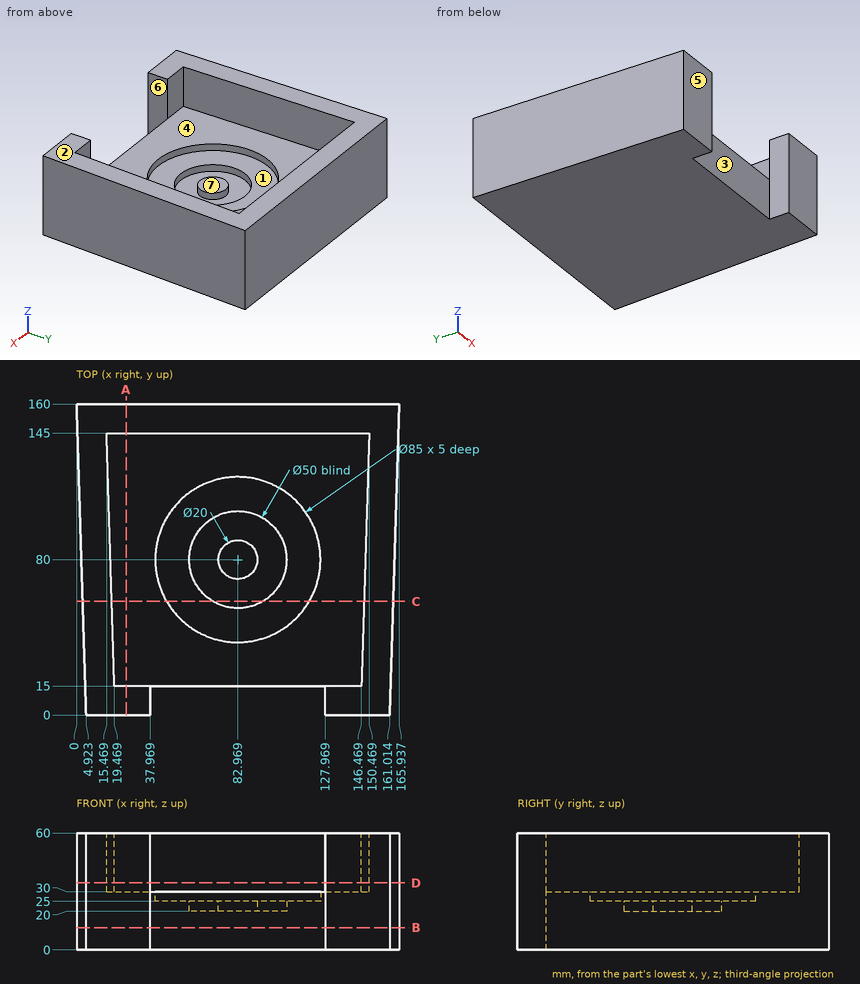
Can you work these out from the drawing? Everything is in mm from the part's minimum corner. A direction names the side the tool comes from. Coordinates: 2 decimals unless noted, no trailing zeros. Loops run counter-clockwise (first coordinate to the right, second up) from the corner with the lowest first, then second, coordinate; pieces in that order, holes last. Notation, with made-up numbers: (54, 83) -> (104, 83) arc R26 ccw to (104, 101) -> close; hole circle Ø6 at (0.5, 7). An arc over 180 degrees is marked (long way). Return JSON: item names as keys, results as strings.
1) If we section it at D-D, the plane z = 34.5: Write out the boundary of the cut face in (x, y), then the cut area to 3 significant figures.
Results below:
{"outline": "(0, 160) -> (4.92, 0) -> (37.97, 0) -> (37.97, 15) -> (19.47, 15) -> (15.47, 145) -> (150.47, 145) -> (146.47, 15) -> (127.97, 15) -> (127.97, 0) -> (161.01, 0) -> (165.94, 160) -> close", "area": "7,380 mm²"}
2) For the marked faces 1, 2 and 3, which set-ups out of +Z, -Z, +X, -X, +Y, -Y let a thin tool reach every point of the face, with its end or its side?
Results below:
{"face 1": "+Z", "face 2": "+Z, +X, -X, +Y, -Y", "face 3": "+Z, -Z, -Y"}
3) Will these pins go through, and if not, where does the flat tip stop? pin 1 (15 mm diameter, centred on x = 72.5, z = 46.5, fed in from -Y); pin 2 (4.5 mm diameter, centred on y = 8.5, z = 21.5, fed in from -X); pin 3 (3 mm diameter, centred on x = 69, y = 122.5, fed in from +Z).
Results below:
{"pin 1": "y = 145", "pin 2": "x = 4.59", "pin 3": "z = 30"}
4) I need wall thicknesses on line 1 (X direction, y = 80, z = 21) (1 decimal); line 2 (Z direction, x = 29.5, y = 106); line 3 (Z direction, x = 73, y = 94.5). Which ranges of each line are inside material? Lowest first, please. Write a range as from..to.
Results below:
{"line 1": "2.5..58, 73..93, 108..163.5", "line 2": "0..30", "line 3": "0..20"}
5) If we section it at C-C, the plane y = 58.5: Write out the boundary of the cut face in (x, z).
Results below:
{"outline": "(3.12, 0) -> (162.81, 0) -> (162.81, 60) -> (147.81, 60) -> (147.81, 30) -> (119.63, 30) -> (119.63, 25) -> (95.73, 25) -> (95.73, 20) -> (70.21, 20) -> (70.21, 25) -> (46.31, 25) -> (46.31, 30) -> (18.13, 30) -> (18.13, 60) -> (3.12, 60) -> close"}
6) If we section it at B-B, the plane z = 11.5: Write out the boundary of the cut face in (x, y).
Results below:
{"outline": "(0, 160) -> (4.92, 0) -> (37.97, 0) -> (37.97, 15) -> (127.97, 15) -> (127.97, 0) -> (161.01, 0) -> (165.94, 160) -> close"}
7) If we section it at A-A, the plane x = 25.5: Write out the boundary of the cut face in (y, z).
Results below:
{"outline": "(0, 0) -> (160, 0) -> (160, 60) -> (145, 60) -> (145, 30) -> (15, 30) -> (15, 60) -> (0, 60) -> close"}
8) Thinking about a two-plate mould opening in Y: for the marked faces 4, 5, 6 and 7, which applies, +Y half, -Y half, draft (parallel to the pull), parting line (faces both ways), or undercut?
Results below:
{"face 4": "undercut", "face 5": "-Y half", "face 6": "draft", "face 7": "undercut"}
